Verification items for this drawing (mm, ordinates from the low corner). A direction names the side the tool comes from. Round coordinates to 2 decimals unless told otherwise and drop trailing zeros. Order: outer loops, then holes, each group sorted by start corner. A loop starts at its lowest first (then second) coordinate and runs counter-clockwise, first axis right, second up.
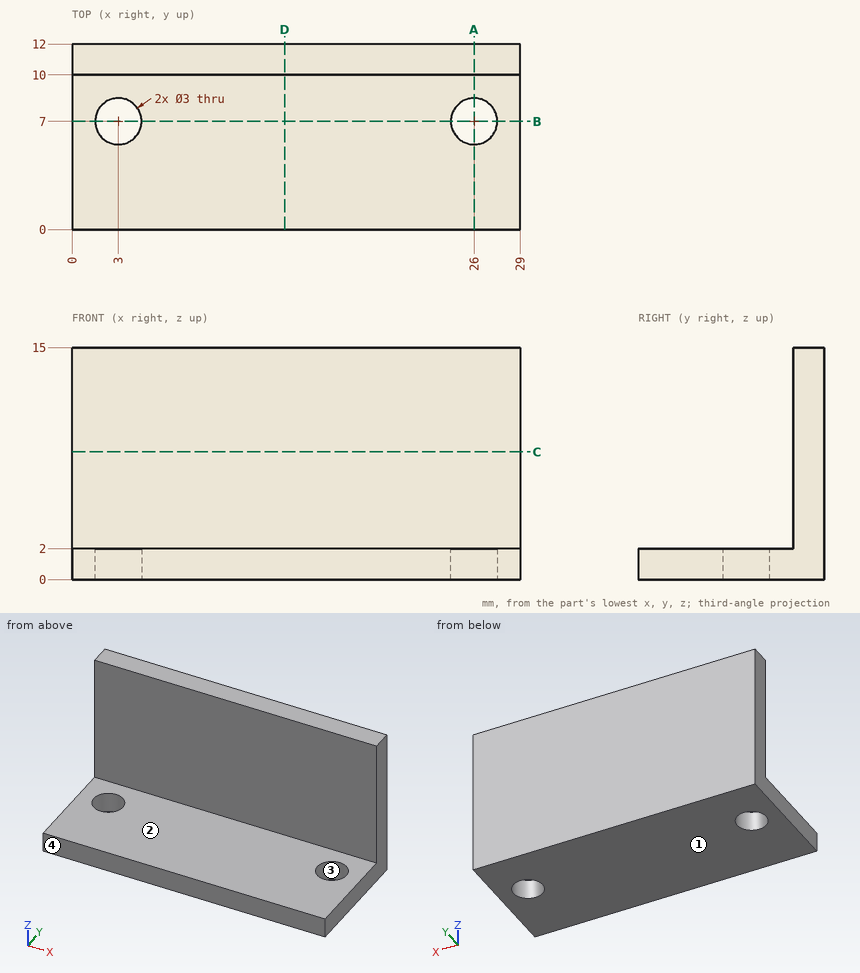
Item 1: Access from +Z, -Z, +X, -X, +Y, -Y to the whole of each face (thin tool, end or side, straight path). Record for the marked faces 1 and 2.
Answer:
face 1: -Z, +X, -X, +Y, -Y
face 2: +Z, +X, -X, -Y
Item 2: Sectioned sample at D-D (x = 13.75). Record the cut outline in (y, z).
Answer:
outline: (0, 0) - (12, 0) - (12, 15) - (10, 15) - (10, 2) - (0, 2) - close
Item 3: Scan lines: line 1 along Y through (x, z) = (3, 0.7); line 2 along Z through (x, y) = (26.25, 3.5); line 3 along Y through (x, z) = (26.25, 8). Record each from-to range of solid material in increasing order.
Answer:
line 1: y = 0 to 5.5, 8.5 to 12
line 2: z = 0 to 2
line 3: y = 10 to 12
Item 4: Go/stop test with flat-tipped pins: P1, Ø2, axis at x = 7, z = 8, coming from the -Y side; P2, Ø4, axis at x = 3, y = 7, coming from the -Z side; P3, Ø6, axis at y = 2, z = 6.5, coming from the +X side. Record where each tip stops, or that it passes through.
Answer:
P1: stops at y = 10
P2: stops at z = 0
P3: passes through
Item 5: Release check for a two-part mould opening along X. For the marked faces 3 and 4 record: released by +X, released by -X, zero draft, split by the parting line, or undercut.
Answer:
face 3: undercut
face 4: zero draft
Item 6: Sectioned sample at A-A (x = 26). Record the cut outline in (y, z), and give its area (3 significant figures).
Answer:
outline: (0, 0) - (5.5, 0) - (5.5, 2) - (0, 2) - close; (8.5, 0) - (12, 0) - (12, 15) - (10, 15) - (10, 2) - (8.5, 2) - close
area: 44.0 mm2
Item 7: Sectioned sample at B-B (y = 7). Record the cut outline in (x, z), and give its area (3 significant figures).
Answer:
outline: (0, 0) - (1.5, 0) - (1.5, 2) - (0, 2) - close; (4.5, 0) - (24.5, 0) - (24.5, 2) - (4.5, 2) - close; (27.5, 0) - (29, 0) - (29, 2) - (27.5, 2) - close
area: 46.0 mm2
Item 8: Sectioned sample at C-C (z = 8.25). Record the cut outline in (x, y), and give its area (3 significant figures).
Answer:
outline: (0, 10) - (29, 10) - (29, 12) - (0, 12) - close
area: 58.0 mm2
